from build123d import *

# Parameters (mm, degrees)
F0_R     = 42.600351
F1_DEPTH = 10
F2_R     = 3
F3_DEPTH = 10
F4_R     = 1.75
F5_DEPTH = 10


with BuildPart() as f1:
    # F0 (on Top) → F1 (new body)
    with BuildSketch(Plane.XY):
        with Locations((-3.491996, 3.379424)):
            Circle(F0_R)
        with BuildLine():
            ThreePointArc((-7.164283, -34.028625), (-15.375556, -32.280481), (-22.994009, -28.753415))
            Line((-22.994009, -28.753415), (-16.57502, -18.424874))
            Line((-16.57502, -18.424874), (-7.164283, -34.028625))
        make_face(mode=Mode.SUBTRACT)
        with BuildLine():
            ThreePointArc((-26.719134, -26.173036), (-36.194012, -15.152333), (-40.779743, -1.361021))
            Line((-40.779743, -1.361021), (-26.045103, -1.361021))
            Line((-26.045103, -1.361021), (-19.285653, -12.996144))
            Line((-19.285653, -12.996144), (-26.719134, -26.173036))
        make_face(mode=Mode.SUBTRACT)
        Polygon((-4.45611, -30.667817), (-33.544526, 19.741029), (-20.909635, 12.940229), (-4.45611, -15.572951), align=None, mode=Mode.SUBTRACT)
        Polygon((-3.691398, -11.018276), (-16.418712, 11.037555), (9.128165, 11.037555), align=None, mode=Mode.SUBTRACT)
        with BuildLine():
            ThreePointArc((16.165116, -28.658769), (8.54654, -32.228461), (0.324819, -34.014155))
            Line((0.324819, -34.014155), (9.573368, -18.149028))
            Line((9.573368, -18.149028), (16.165116, -28.658769))
        make_face(mode=Mode.SUBTRACT)
        Polygon((-2.912057, -15.508026), (14.16059, 12.940229), (26.090452, 19.84215), (-2.912057, -30.488131), align=None, mode=Mode.SUBTRACT)
        with BuildLine():
            Line((19.884041, -26.055397), (12.450778, -12.686017))
            Line((12.450778, -12.686017), (18.892192, -1.584855))
            Line((18.892192, -1.584855), (33.766611, -1.584855))
            ThreePointArc((33.766611, -1.584855), (29.201151, -15.167973), (19.884041, -26.055397))
        make_face(mode=Mode.SUBTRACT)
        with BuildLine():
            ThreePointArc((-41.071032, 2.564623), (-40.341471, 10.793199), (-37.83205, 18.663683))
            Line((-37.83205, 18.663683), (-28.703782, 2.564623))
            Line((-28.703782, 2.564623), (-41.071032, 2.564623))
        make_face(mode=Mode.SUBTRACT)
        Polygon((-20.089835, 13.989503), (-32.347553, 21.261031), (25.130622, 21.261031), (13.177481, 13.989503), align=None, mode=Mode.SUBTRACT)
        with BuildLine():
            Line((-16.344654, 25.73009), (-33.712777, 25.73009))
            ThreePointArc((-33.712777, 25.73009), (-28.452661, 31.483037), (-22.119012, 36.027275))
            Line((-22.119012, 36.027275), (-16.344654, 25.73009))
        make_face(mode=Mode.SUBTRACT)
        with BuildLine():
            Line((-10.259116, 25.144359), (-17.628212, 38.207793))
            ThreePointArc((-17.628212, 38.207793), (-3.588235, 40.96717), (10.465687, 38.279725))
            Line((10.465687, 38.279725), (3.075884, 25.144359))
            Line((3.075884, 25.144359), (-10.259116, 25.144359))
        make_face(mode=Mode.SUBTRACT)
        with BuildLine():
            ThreePointArc((30.767179, 18.844119), (33.358844, 10.786409), (34.081858, 2.353102))
            Line((34.081858, 2.353102), (21.473352, 2.353102))
            Line((21.473352, 2.353102), (30.767179, 18.844119))
        make_face(mode=Mode.SUBTRACT)
        with BuildLine():
            ThreePointArc((14.803284, 36.214323), (21.354359, 31.584149), (26.773684, 25.669252))
            Line((26.773684, 25.669252), (8.578651, 25.669252))
            Line((8.578651, 25.669252), (14.803284, 36.214323))
        make_face(mode=Mode.SUBTRACT)
    extrude(amount=F1_DEPTH)

    # F2 (on face) → F3 (join, through all)
    with BuildSketch(Plane.XY.offset(10)):
        with Locations((-3.588235, 45.396723)):
            Circle(F2_R)
    extrude(amount=-F3_DEPTH)

    # F4 (on face) → F5 (cut, through all)
    with BuildSketch(Plane.XY.offset(10)):
        with Locations((-3.588235, 45.396723)):
            Circle(F4_R)
    extrude(amount=-F5_DEPTH, mode=Mode.SUBTRACT)


solid = f1.part
Read the model definition and answer for the solid it produces. Units are mm, in the model's axes. Round coordinates to 2 decimals unless told otherwise and drop trailing zeros. Write each loop counter-clockwise with the first axis right and the second up, starting at its lowest first coordinate (ties: lowest second). Pieces come first, ordered by that corner, then holes.
Q1. Find section A-A on y = -24. Determine the outline of the cut face in (x, z).
Values:
outline: (-36.13, 0) - (-29.24, 0) - (-29.24, 10) - (-36.13, 10) - close; (-25.49, 0) - (-20.04, 0) - (-20.04, 10) - (-25.49, 10) - close; (-13.21, 0) - (-8.3, 0) - (-8.3, 10) - (-13.21, 10) - close; (-4.46, 0) - (-2.91, 0) - (-2.91, 10) - (-4.46, 10) - close; (0.83, 0) - (6.16, 0) - (6.16, 10) - (0.83, 10) - close; (13.24, 0) - (18.74, 0) - (18.74, 10) - (13.24, 10) - close; (22.26, 0) - (29.14, 0) - (29.14, 10) - (22.26, 10) - close
Q2. Flat-ended cylindrical pins translate along their axes: P1, Ø5, axis at x = 28.5, z = 5, coming from the +Y side; P2, Ø5, axis at x = -34, z = 5.5, coming from the -Y side; P3, Ø2, axis at y = 20.5, z = 1.5, coming from the -X side; P4, Ø6, axis at x = -1, y = -18.5, coming from the +Z side. Find the tip coordinate at first contact, or state that the pin passes through.
Values:
P1: stops at y = 34.12
P2: stops at y = -28.72
P3: stops at x = -42.92
P4: stops at z = 10
Q3. The mould has two halves that part along X. Classify faces 1 (the face through (-14, 5, 10)), 2 (the face through (-4, 11.038, 5)), 3 (the face through (-3.536, 48.396, 5.07)): released by +X, released by -X, zero draft, split by the parting line, or undercut.
Values:
face 1: zero draft
face 2: undercut
face 3: split by the parting line
Q4. Find section B-B on x = 1.5. Determine the outline of the cut face in (y, z), and give its area (3 significant figures).
Values:
outline: (-38.93, 0) - (-33.88, 0) - (-33.88, 10) - (-38.93, 10) - close; (-32, 0) - (-22.83, 0) - (-22.83, 10) - (-32, 10) - close; (-8.16, 0) - (-2.09, 0) - (-2.09, 10) - (-8.16, 10) - close; (11.04, 0) - (13.99, 0) - (13.99, 10) - (11.04, 10) - close; (21.26, 0) - (25.14, 0) - (25.14, 10) - (21.26, 10) - close; (40.63, 0) - (45.69, 0) - (45.69, 10) - (40.63, 10) - close
area: 322 mm2
Q5. Find section C-C on x = -36.5. Determine the outline of the cut face in (y, z).
Values:
outline: (-23.55, 0) - (-14.6, 0) - (-14.6, 10) - (-23.55, 10) - close; (-1.36, 0) - (2.56, 0) - (2.56, 10) - (-1.36, 10) - close; (16.31, 0) - (30.31, 0) - (30.31, 10) - (16.31, 10) - close
Q6. Straight lines are drawn through the part: line 1 (Y direction, x = 20.5, z = 3); line 2 (Y direction, x = -15, z = 8.25); line 3 (X direction, y = 15.5, z = 1.5). For each, find the intervals that lie inside material, in ascending order.
Values:
line 1: y = -31.82 to -25.56, -1.58 to 10.14, 16.61 to 18.44, 21.26 to 25.67, 32.31 to 38.58
line 2: y = -37.64 to -32.4, -21.04 to -12.4, 2.7 to 8.58, 11.04 to 13.99, 21.26 to 33.55, 39.16 to 44.4
line 3: x = -44.33 to -39.07, -36.04 to -31.1, -25.67 to -22.64, 15.66 to 18.59, 23.59 to 28.88, 32.09 to 37.35
Q7. Find section D-D on y = -14. Determine the outline of the cut face in (x, z).
Values:
outline: (-42.39, 0) - (-36.82, 0) - (-36.82, 10) - (-42.39, 10) - close; (-19.85, 0) - (-14.07, 0) - (-14.07, 10) - (-19.85, 10) - close; (-5.36, 0) - (-2.01, 0) - (-2.01, 10) - (-5.36, 10) - close; (6.59, 0) - (13.18, 0) - (13.18, 10) - (6.59, 10) - close; (29.84, 0) - (35.4, 0) - (35.4, 10) - (29.84, 10) - close
